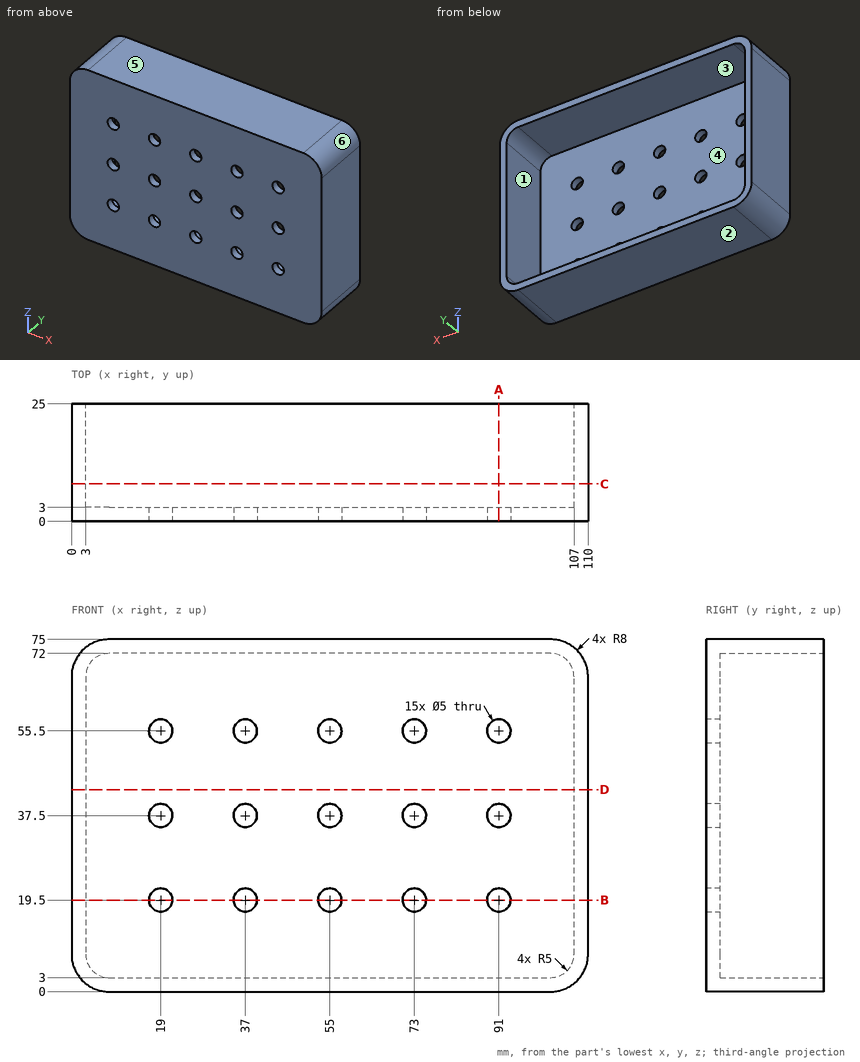
Here's the drawing with two shaded views (mm, measured from the low corner). I have some questions. A direction names the side the tool comes from. Coordinates: 2 decimals unless noted, no trailing zeros. Write each loop counter-clockwise with the first axis right and the second up, starting at its lowest first coordinate (ties: lowest second). Pieces come first, ordered by that corner, then holes. Notation, with made-up numbers: (-27, 21) -> (-4, 21) arc R20 cw to (-4, 38) -> close; hole circle Ø6 at (65, -3). An arc over 180 degrees is marked (long way). Use a Markdown table: item, result. Add a question column.
(1) We'd pull the mould along X, two halves only. Please class the marked faces 3, 4, 5 and 6: +X half, -X half, draft (parallel to the pull), parting line (faces both ways), or undercut.
(2) If we section it at D-D, the plane z = 43: Write out the boundary of the cut face in (x, y).
(3) If we section it at C-C, the plane y = 8: Write out the boundary of the cut face in (x, z).
(4) For the marked faces 1 and 2, which set-ups out of +Z, -Z, +X, -X, +Y, -Y let a thin tool reach every point of the face, with its end or its side?
(5) If we section it at A-A, the plane x = 91: Write out the boundary of the cut face in (y, z), and give its area (3 significant figures).
(6) Please list where these lines run through material, in increasing order: line 1 (X direction, y = 1.6, z = 19.5); line 2 (Z direction, x = 91, y = 0.9); line 3 (Z direction, x = 43, y = 9.75).
(7) I'm going to push a flat-ended pin straight in: P1, Ø1.5, axis at x = 27.5, z = 48, coming from the +Y side. Where does the tip first touch, or does it pass through?
(8) If we section it at B-B, the plane z = 19.5: Write out the boundary of the cut face in (x, y), and give its area (3 significant figures).
Outcome:
| question | item | result |
|---|---|---|
| 1 | face 3 | undercut |
| 1 | face 4 | undercut |
| 1 | face 5 | draft |
| 1 | face 6 | +X half |
| 2 | outline | (0, 0) -> (110, 0) -> (110, 25) -> (107, 25) -> (107, 3) -> (3, 3) -> (3, 25) -> (0, 25) -> close |
| 3 | outline | (0, 8) arc R8 ccw to (8, 0) -> (102, 0) arc R8 ccw to (110, 8) -> (110, 67) arc R8 ccw to (102, 75) -> (8, 75) arc R8 ccw to (0, 67) -> close; hole (3, 8) arc R5 ccw to (8, 3) -> (102, 3) arc R5 ccw to (107, 8) -> (107, 67) arc R5 ccw to (102, 72) -> (8, 72) arc R5 ccw to (3, 67) -> close |
| 4 | face 1 | +Y |
| 4 | face 2 | -Z, +X, -X, +Y, -Y |
| 5 | outline | (0, 0) -> (25, 0) -> (25, 3) -> (3, 3) -> (3, 17) -> (0, 17) -> close; (0, 22) -> (3, 22) -> (3, 35) -> (0, 35) -> close; (0, 40) -> (3, 40) -> (3, 53) -> (0, 53) -> close; (0, 58) -> (3, 58) -> (3, 72) -> (25, 72) -> (25, 75) -> (0, 75) -> close |
| 5 | area | 312 mm^2 |
| 6 | line 1 | x = 0 to 16.5, 21.5 to 34.5, 39.5 to 52.5, 57.5 to 70.5, 75.5 to 88.5, 93.5 to 110 |
| 6 | line 2 | z = 0 to 17, 22 to 35, 40 to 53, 58 to 75 |
| 6 | line 3 | z = 0 to 3, 72 to 75 |
| 7 | P1 | stops at y = 3 |
| 8 | outline | (0, 0) -> (16.5, 0) -> (16.5, 3) -> (3, 3) -> (3, 25) -> (0, 25) -> close; (21.5, 0) -> (34.5, 0) -> (34.5, 3) -> (21.5, 3) -> close; (39.5, 0) -> (52.5, 0) -> (52.5, 3) -> (39.5, 3) -> close; (57.5, 0) -> (70.5, 0) -> (70.5, 3) -> (57.5, 3) -> close; (75.5, 0) -> (88.5, 0) -> (88.5, 3) -> (75.5, 3) -> close; (93.5, 0) -> (110, 0) -> (110, 25) -> (107, 25) -> (107, 3) -> (93.5, 3) -> close |
| 8 | area | 387 mm^2 |
